from build123d import *

# Parameters (mm, degrees)
SKETCH1_W                      = 19
SKETCH1_H                      = 19
SKETCH1_W_2                    = 15.875
SKETCH1_H_2                    = 15.875
TUBE_DEPTH                     = 758.9266
SKETCH2_R                      = 2.8956
SIDE_WALL_HOLES_DEPTH          = 20
LPATTERN1_COUNT                = 4
LPATTERN1_PITCH                = 234.974466667
CUT_EXTRUDE1_REACH             = 21
SKETCH3_R                      = 4.7625
CUT_EXTRUDE1_DIRECTION_2_DEPTH = 1


with BuildPart() as part:
    # Sketch1 → Tube (new body)
    with BuildSketch(Plane(origin=(0, 0, 0), x_dir=(1, 0, 0), z_dir=(0, 1, 0))):
        Rectangle(SKETCH1_W, SKETCH1_H)
        Rectangle(SKETCH1_W_2, SKETCH1_H_2, mode=Mode.SUBTRACT)
    extrude(amount=TUBE_DEPTH)

    # Sketch2 → Side Wall Holes (cut, through all)
    with BuildSketch(Plane.XY.offset(9.5)):
        with Locations((0, 731.925)):
            Circle(SKETCH2_R)
    side_wall_holes = extrude(amount=-SIDE_WALL_HOLES_DEPTH, mode=Mode.SUBTRACT)

    # LPattern1: Side Wall Holes ×4
    with Locations(*[(0, -i * LPATTERN1_PITCH, 0) for i in range(1, LPATTERN1_COUNT)]):
        add(side_wall_holes, mode=Mode.SUBTRACT)

    # Sketch3 → Cut-Extrude1 (cut, up to next)
    with BuildSketch(Plane.ZY.offset(9.5), mode=Mode.PRIVATE) as cut_extrude1_sk1:
        with Locations((0, 674.37)):
            Circle(SKETCH3_R)
    cut_extrude1_tool1 = extrude(cut_extrude1_sk1.sketch, amount=-CUT_EXTRUDE1_REACH, mode=Mode.PRIVATE) & part.part
    add(cut_extrude1_tool1.solids().sort_by_distance((-9.5, 674.37, 0))[0], mode=Mode.SUBTRACT)
    # Sketch3 → Cut-Extrude1 (cut, up to next)
    with BuildSketch(Plane.ZY.offset(9.5), mode=Mode.PRIVATE) as cut_extrude1_sk2:
        with Locations((0, 84.5566)):
            Circle(SKETCH3_R)
    cut_extrude1_tool2 = extrude(cut_extrude1_sk2.sketch, amount=-CUT_EXTRUDE1_REACH, mode=Mode.PRIVATE) & part.part
    add(cut_extrude1_tool2.solids().sort_by_distance((-9.5, 84.5566, 0))[0], mode=Mode.SUBTRACT)

    # Sketch3 → Cut-Extrude1 direction 2 (cut)
    with BuildSketch(Plane.ZY.offset(9.5)):
        with Locations((0, 674.37)):
            Circle(SKETCH3_R)
        with Locations((0, 84.5566)):
            Circle(SKETCH3_R)
    extrude(amount=CUT_EXTRUDE1_DIRECTION_2_DEPTH, mode=Mode.SUBTRACT)


solid = part.part
Design review of the part built by this model. Coordinates are the model's own, in mm. A direction names the side the tool comes from. Coordinates: 2 decimals unless noted, no trailing zeros. Loops run counter-clockwise (first coordinate to the right, second up) from the corner with the lowest first, then second, coordinate; pieces in that order, holes last. Notation, with made-up numbers: M 18,8.25 L 74,8.25 A20 cw 74,12.25 Z; hole C 55,38.5 d6. An arc over 180 degrees is marked long. Answer as CSV lines item,"result".
Item 1: Add section C-C on x = 0. Count the separate pieces of the cut face and the enclosed holes in it, plus the area to 3 significant figures.
Answer list:
separate pieces,"10"
enclosed holes,"0"
area,"2,300 mm²"
Item 2: Machinability: for faces 1 (the face through (0, 374, -7.938)), 2 (the face through (-9.5, 374, 0)), which of the approach directions +Z, -Z, +X, -X, +Y, -Y give a long, thin tool a straight path to every point of the face, cutting with its end or side? Answer none if there is none.
Answer list:
face 1,"+Y, -Y"
face 2,"+Z, -Z, -X, +Y, -Y"
Item 3: Add section A-A on z = 0. State the section outline as (x, y) points.
Answer list:
outline,"M -9.5,0 L -7.94,0 L -7.94,79.79 L -9.5,79.79 Z; M -9.5,89.32 L -7.94,89.32 L -7.94,669.61 L -9.5,669.61 Z; M -9.5,679.13 L -7.94,679.13 L -7.94,758.93 L -9.5,758.93 Z; M 7.94,0 L 9.5,0 L 9.5,758.93 L 7.94,758.93 Z"
Item 4: The part is to be moulded in two halves that separate along Z. For faces 3 (the face through (0, 374, 7.938)), 4 (the face through (0, 374, -9.5)), 5 (the face through (0, 374, 9.5)), say which applies: pulls with the +Z half, pulls with the -Z half, needs draft (parallel to the pull), parting line crosses it, or undercut.
Answer list:
face 3,"undercut"
face 4,"pulls with the -Z half"
face 5,"pulls with the +Z half"
Item 5: For probe 1 along Y at (x, z) = (0, -9.15); probe 2 along X at (y, z) = (204, -7); probe 3 along Z at (x, y) = (-9.05, 674.37), list the stretches that pass through material, from the lowest coordinate up.
Answer list:
probe 1,"0 to 24.11, 29.9 to 259.08, 264.87 to 494.05, 499.85 to 729.03, 734.82 to 758.93"
probe 2,"-9.5 to -7.94, 7.94 to 9.5"
probe 3,"-9.5 to -4.76, 4.76 to 9.5"
Item 6: Add section B-B on y = 212. State the section outline as (x, z) points, plus the area to 3 significant figures.
Answer list:
outline,"M -9.5,-9.5 L 9.5,-9.5 L 9.5,9.5 L -9.5,9.5 Z; hole M -7.94,-7.94 L 7.94,-7.94 L 7.94,7.94 L -7.94,7.94 Z"
area,"109 mm²"
